from build123d import *

# Parameters (mm, degrees)
F1_DEPTH  = 15.748
F2_R      = 34.925
F3_DEPTH  = 38.1
F4_R      = 23.876
F5_DEPTH  = 38.1
F6_R      = 23.876
F7_DEPTH  = 38.1
F9_DEPTH  = 50.8
F10_R     = 28.575
F10_R_2   = 23.876
F11_DEPTH = 35.052


with BuildPart() as f1:
    # F0 (on Front) → F1 (new body)
    with BuildSketch(Plane.XZ):
        with BuildLine():
            Line((35.867186, -23.583606), (38.19529, -19.589827))
            ThreePointArc((38.19529, -19.589827), (41.726565, -10.076469), (42.926, 0))
            ThreePointArc((42.926, 0), (41.43258, 11.224206), (37.056234, 21.667419))
            ThreePointArc((37.056234, 21.667419), (25.604433, 34.453657), (10.058576, 41.730882))
            ThreePointArc((10.058576, 41.730882), (5.346921, 39.035507), (0, 38.1))
            Line((0, 38.1), (0, 0))
            Line((0, 0), (0, -38.1))
            ThreePointArc((0, -38.1), (5.346921, -39.035507), (10.058576, -41.730882))
            ThreePointArc((10.058576, -41.730882), (24.690581, -35.114337), (35.867186, -23.583606))
        make_face()
        with BuildLine():
            ThreePointArc((35.867186, -23.583606), (37.085039, -21.618079), (38.19529, -19.589827))
            Line((38.19529, -19.589827), (35.867186, -23.583606))
        make_face()
        with BuildLine():
            Line((13.752612, -61.520364), (35.867186, -23.583606))
            ThreePointArc((35.867186, -23.583606), (24.690581, -35.114337), (10.058576, -41.730882))
            ThreePointArc((10.058576, -41.730882), (14.254858, -47.15483), (15.748, -53.848))
            ThreePointArc((15.748, -53.848), (15.240991, -57.811797), (13.752612, -61.520364))
        make_face()
        with BuildLine():
            ThreePointArc((10.058576, 41.730882), (25.604433, 34.453657), (37.056234, 21.667419))
            Line((37.056234, 21.667419), (13.73214, 61.556945))
            ThreePointArc((13.73214, 61.556945), (15.235702, 57.832078), (15.748, 53.848))
            ThreePointArc((15.748, 53.848), (14.254858, 47.15483), (10.058576, 41.730882))
        make_face()
        with BuildLine():
            ThreePointArc((6.604, -53.848), (4.669733, -49.178267), (0, -47.244))
            ThreePointArc((0, -47.244), (-4.669733, -58.517733), (6.604, -53.848))
        make_face()
        with BuildLine():
            ThreePointArc((15.748, -53.848), (14.254858, -47.15483), (10.058576, -41.730882))
            ThreePointArc((10.058576, -41.730882), (5.064663, -42.626173), (0, -42.926))
            ThreePointArc((0, -42.926), (-5.064663, -42.626173), (-10.058576, -41.730882))
            ThreePointArc((-10.058576, -41.730882), (-15.484435, -50.978895), (-13.73214, -61.556945))
            Line((-13.73214, -61.556945), (-13.452853, -62.034589))
            ThreePointArc((-13.452853, -62.034589), (0, -69.596), (13.452853, -62.034589))
            Line((13.452853, -62.034589), (13.752612, -61.520364))
            ThreePointArc((13.752612, -61.520364), (15.240991, -57.811797), (15.748, -53.848))
        make_face()
        with BuildLine():
            ThreePointArc((6.604, -53.848), (-4.669733, -58.517733), (0, -47.244))
            ThreePointArc((0, -47.244), (4.669733, -49.178267), (6.604, -53.848))
        make_face(mode=Mode.SUBTRACT)
        with BuildLine():
            ThreePointArc((13.452853, -62.034589), (13.605162, -61.778893), (13.752612, -61.520364))
            Line((13.752612, -61.520364), (13.452853, -62.034589))
        make_face()
        with BuildLine():
            ThreePointArc((6.604, 53.848), (-4.669733, 58.517733), (0, 47.244))
            ThreePointArc((0, 47.244), (4.669733, 49.178267), (6.604, 53.848))
        make_face()
        with BuildLine():
            ThreePointArc((0, 42.926), (5.064663, 42.626173), (10.058576, 41.730882))
            ThreePointArc((10.058576, 41.730882), (14.254858, 47.15483), (15.748, 53.848))
            ThreePointArc((15.748, 53.848), (15.235702, 57.832078), (13.73214, 61.556945))
            Line((13.73214, 61.556945), (13.452853, 62.034589))
            ThreePointArc((13.452853, 62.034589), (0, 69.596), (-13.452853, 62.034589))
            Line((-13.452853, 62.034589), (-13.755504, 61.515177))
            ThreePointArc((-13.755504, 61.515177), (-15.480058, 50.955369), (-10.058576, 41.730882))
            ThreePointArc((-10.058576, 41.730882), (-5.064663, 42.626173), (0, 42.926))
        make_face()
        with BuildLine():
            ThreePointArc((6.604, 53.848), (4.669733, 49.178267), (0, 47.244))
            ThreePointArc((0, 47.244), (-4.669733, 58.517733), (6.604, 53.848))
        make_face(mode=Mode.SUBTRACT)
        with BuildLine():
            Line((13.452853, 62.034589), (13.73214, 61.556945))
            ThreePointArc((13.73214, 61.556945), (13.594595, 61.796994), (13.452853, 62.034589))
        make_face()
        with BuildLine():
            ThreePointArc((-10.058576, -41.730882), (-5.346921, -39.035507), (0, -38.1))
            Line((0, -38.1), (0, 0))
            Line((0, 0), (0, 38.1))
            ThreePointArc((0, 38.1), (-5.346921, 39.035507), (-10.058576, 41.730882))
            ThreePointArc((-10.058576, 41.730882), (-24.629018, 35.157545), (-35.784322, 23.70915))
            Line((-35.784322, 23.70915), (-38.271037, 19.441429))
            ThreePointArc((-38.271037, 19.441429), (-42.90727, -1.267948), (-37.056234, -21.667418))
            ThreePointArc((-37.056234, -21.667418), (-25.604433, -34.453657), (-10.058576, -41.730882))
        make_face()
        with BuildLine():
            ThreePointArc((-13.73214, -61.556945), (-15.484435, -50.978895), (-10.058576, -41.730882))
            ThreePointArc((-10.058576, -41.730882), (-25.604433, -34.453657), (-37.056234, -21.667418))
            Line((-37.056234, -21.667418), (-13.73214, -61.556945))
        make_face()
        with BuildLine():
            ThreePointArc((-13.73214, -61.556945), (-13.594595, -61.796994), (-13.452853, -62.034589))
            Line((-13.452853, -62.034589), (-13.73214, -61.556945))
        make_face()
        with BuildLine():
            ThreePointArc((-35.784322, 23.70915), (-24.629018, 35.157545), (-10.058576, 41.730882))
            ThreePointArc((-10.058576, 41.730882), (-15.480058, 50.955369), (-13.755504, 61.515177))
            Line((-13.755504, 61.515177), (-35.784322, 23.70915))
        make_face()
        with BuildLine():
            Line((-13.755504, 61.515177), (-13.452853, 62.034589))
            ThreePointArc((-13.452853, 62.034589), (-13.606657, 61.776328), (-13.755504, 61.515177))
        make_face()
        with BuildLine():
            Line((-38.271037, 19.441429), (-35.784322, 23.70915))
            ThreePointArc((-35.784322, 23.70915), (-37.089114, 21.611087), (-38.271037, 19.441429))
        make_face()
        with BuildLine():
            ThreePointArc((0, 38.1), (5.346921, 39.035507), (10.058576, 41.730882))
            ThreePointArc((10.058576, 41.730882), (5.064663, 42.626173), (0, 42.926))
            Line((0, 42.926), (0, 38.1))
        make_face()
        with BuildLine():
            Line((0, 38.1), (0, 42.926))
            ThreePointArc((0, 42.926), (-5.064663, 42.626173), (-10.058576, 41.730882))
            ThreePointArc((-10.058576, 41.730882), (-5.346921, 39.035507), (0, 38.1))
        make_face()
        with BuildLine():
            ThreePointArc((0, -42.926), (5.064663, -42.626173), (10.058576, -41.730882))
            ThreePointArc((10.058576, -41.730882), (5.346921, -39.035507), (0, -38.1))
            Line((0, -38.1), (0, -42.926))
        make_face()
        with BuildLine():
            ThreePointArc((-10.058576, -41.730882), (-5.064663, -42.626173), (0, -42.926))
            Line((0, -42.926), (0, -38.1))
            ThreePointArc((0, -38.1), (-5.346921, -39.035507), (-10.058576, -41.730882))
        make_face()
    extrude(amount=F1_DEPTH)

    # F2 (on face) → F3 (join)
    with BuildSketch(Plane.XZ.offset(15.748)):
        Circle(F2_R)
    extrude(amount=-F3_DEPTH)

    # F4 (on face) → F5 (join)
    with BuildSketch(Plane.XZ.offset(15.748)):
        Circle(F4_R)
    extrude(amount=-F5_DEPTH)

    # F6 (on face) → F7 (cut)
    with BuildSketch(Plane.XZ.offset(15.748)):
        Circle(F6_R)
    extrude(amount=-F7_DEPTH, mode=Mode.SUBTRACT)

    # F8 (on Right) → F9 (cut)
    with BuildSketch(Plane.YZ):
        with BuildLine():
            Line((-7.874, 6.604), (-7.874, 0))
            Line((-7.874, 0), (-7.874, -6.604))
            ThreePointArc((-7.874, -6.604), (-5.75692, -7.459222), (-4.82788, -9.544963))
            Line((-4.82788, -9.544963), (-4.82788, 9.544963))
            ThreePointArc((-4.82788, 9.544963), (-5.75692, 7.459222), (-7.874, 6.604))
        make_face()
        with BuildLine():
            Line((-7.874, -6.604), (-7.874, 0))
            Line((-7.874, 0), (-7.874, 6.604))
            ThreePointArc((-7.874, 6.604), (-10.029157, 7.496634), (-10.922, 9.651705))
            Line((-10.922, 9.651705), (-10.920141, -9.545553))
            ThreePointArc((-10.920141, -9.545553), (-9.991292, -7.459427), (-7.874, -6.604))
        make_face()
        with BuildLine():
            ThreePointArc((-4.82788, -9.544963), (-5.75692, -7.459222), (-7.874, -6.604))
            ThreePointArc((-7.874, -6.604), (-9.991292, -7.459427), (-10.920141, -9.545553))
            Line((-10.920141, -9.545553), (-10.92012, -9.759037))
            ThreePointArc((-10.92012, -9.759037), (-7.874, -12.7), (-4.82788, -9.759037))
            Line((-4.82788, -9.759037), (-4.82788, -9.544963))
        make_face()
        with BuildLine():
            ThreePointArc((-10.922, 9.651705), (-10.029157, 7.496634), (-7.874, 6.604))
            ThreePointArc((-7.874, 6.604), (-5.75692, 7.459222), (-4.82788, 9.544963))
            ThreePointArc((-4.82788, 9.544963), (-4.82647, 9.598473), (-4.826, 9.652))
            ThreePointArc((-4.826, 9.652), (-7.874148, 12.7), (-10.922, 9.651705))
        make_face()
        with BuildLine():
            ThreePointArc((-4.826, -9.652), (-4.82647, -9.598473), (-4.82788, -9.544963))
            Line((-4.82788, -9.544963), (-4.82788, -9.759037))
            ThreePointArc((-4.82788, -9.759037), (-4.82647, -9.705527), (-4.826, -9.652))
        make_face()
        with BuildLine():
            Line((-10.92012, -9.759037), (-10.920141, -9.545553))
            ThreePointArc((-10.920141, -9.545553), (-10.922, -9.652295), (-10.92012, -9.759037))
        make_face()
    extrude(amount=F9_DEPTH, mode=Mode.SUBTRACT)

    # F10 (on face) → F11 (cut)
    with BuildSketch(Plane.XZ.offset(15.748)):
        Circle(F10_R)
        Circle(F10_R_2, mode=Mode.SUBTRACT)
    extrude(amount=-F11_DEPTH, mode=Mode.SUBTRACT)


solid = f1.part
Check sheet for the modelled part. Datum: model origin and axes. Units: mm. A direction names the side the tool comes from. Round coordinates to 2 decimals unless told otherwise and drop trailing zeros. Loops run counter-clockwise (first coordinate to the right, second up) from the corner with the lowest first, then second, coordinate; pieces in that order, holes last. Notation, with made-up numbers: (-33.5, 42) -> (4.5, 42) arc R24 ccw to (4.5, 74) -> close; hole circle Ø7 at (85, 37.5). An arc over 180 degrees is marked (long way). Put each result on its own line as item: value. Start each with the question number.
1. Scan lines: probe 1 along Z at (x, y) = (0, -8) (3 decimals); probe 2 along Z at (x, y) = (0, 21.3) (3 decimals); probe 3 along Z at (x, y) = (0, 4) (3 decimals). Record each from-to range of solid material in increasing order.
2. Section check D-D (x = 32.5). Enter the section's corners in (y, z).
3. Section check C-C (y = 9.5). Enter the section's corners in (x, z) (3 decimals).
4. Gauge pin test, flat ends, axial feed: pin 1 (5 mm diameter, centred on y = 10.5, z = -20, fed in from +X); pin 2 (10 mm diameter, centred on x = -11.5, y = 9.5, fed in from +Z); pin 3 (3 mm diameter, centred on x = 16, z = -39, fed in from +Y); pin 4 (10 mm diameter, centred on x = 30, z = -52.5, fed in from +Y). Record the tip position at first contact, or that the pin passes through.
5. Section check B-B (x = 5). Enter the section's corners in (y, z), plus the area to 3 significant figures.
6. Section check A-A (z = 57.5). Enter the section's corners in (x, y), plus the area to 3 significant figures.
7. Access from +Z, -Z, +X, -X, +Y, -Y to the whole of each face (thin tool, end or side, straight path). Record for faces 4 (the face through (0.226, -7.764, 69.594)), 5 (the face through (-27.715, 11.02, -21.251)), 6 (the face through (-28.547, 1.533, 1.256)), 7 (the face through (35, -4.828, 0)).
8. Draft check along Y on faces 1 (the face through (-37.07, -7.76, 21.64)), 2 (the face through (-6.48, 19.304, -23.15)), 3 (the face through (33.6, -7.9, -12.7)). Enter one of: +Y half, -Y half, draft (parallel to the pull), parting line (faces both ways), or undercut.
Findings:
1. probe 1: z = -69.596 to -60.452, -47.244 to -28.575, 28.575 to 47.244, 60.452 to 69.596
1. probe 2: z = -34.925 to -23.876, 23.876 to 34.925
1. probe 3: z = -34.925 to -28.575, 28.575 to 34.925
2. outline: (-15.75, -29.36) -> (0, -29.36) -> (0, -12.79) -> (22.35, -12.79) -> (22.35, 12.79) -> (0, 12.79) -> (0, 29.46) -> (-15.75, 29.46) -> close; hole (-10.92, -9.76) arc R3.05 ccw to (-4.83, -9.76) arc R3.05 ccw to (-4.83, -9.65) arc R3.05 ccw to (-4.83, -9.54) -> (-4.83, 9.54) arc R3.05 ccw to (-4.83, 9.65) arc R3.05 ccw to (-10.92, 9.65) -> (-10.92, -9.55) arc R3.05 ccw to start
3. outline: circle Ø69.85 at (0, 0); hole circle Ø57.15 at (0, 0)
4. pin 1: stops at x = 30.22
4. pin 2: stops at z = 34.31
4. pin 3: stops at y = 0
4. pin 4: passes through
5. outline: (-15.75, -68.78) -> (0, -68.78) -> (0, -58.16) -> (-15.75, -58.16) -> close; (-15.75, -49.53) -> (0, -49.53) -> (0, -34.57) -> (22.35, -34.57) -> (22.35, -23.35) -> (19.3, -23.35) -> (19.3, -28.13) -> (-15.75, -28.13) -> close; (-15.75, 28.13) -> (19.3, 28.13) -> (19.3, 23.35) -> (22.35, 23.35) -> (22.35, 34.57) -> (0, 34.57) -> (0, 49.53) -> (-15.75, 49.53) -> close; (-15.75, 58.16) -> (0, 58.16) -> (0, 68.78) -> (-15.75, 68.78) -> close
5. area: 1,330 mm^2
6. outline: (-16.1, -15.75) -> (-5.5, -15.75) -> (-5.5, 0) -> (-16.1, 0) -> close; (5.5, -15.75) -> (16.1, -15.75) -> (16.1, 0) -> (5.5, 0) -> close
6. area: 334 mm^2
7. face 4: +Z, +Y, -Y
7. face 5: +Y
7. face 6: -Y
7. face 7: +X
8. face 1: draft
8. face 2: -Y half
8. face 3: undercut
